Source: three-view drawing plus pictorial views. Frame: mm from the lowest corner of the part. Give positions to 0.01 mm unless a question says otherwise; leave off trailing zeros. Loops run counter-clockwise (first coordinate to the right, second up) from the corner with the lowest first, then second, coordinate; pieces in that order, holes last. Notation, with made-up numbers: (50, 52) - (101, 52) arc R26 ccw to (101, 91) - close; hole circle Ø8 at (-15.5, -32). An arc over 180 degrees is marked (long way). Answer as a JSON object with one key per item and string values. Group by question number.
(1) Section query B-B (y = 4.3). Return loops of the section in (x, z), plus the area to 3 significant figures.
(2) Material intervals for L1, parallel to X at y = 0.3, z = 2.9; L2, parallel to Z at x = 55, y = 3.1; L3, parallel to Y at x = 57, z = 4.1, sorted ascending.
(3) Mould query, pull axis X, two halves, no side actions, for the marked faces 1, 2, 3 and 4. Classes: +X half, -X half, draft (parallel to the pull), parting line (faces both ways), or undercut.
(4) Pin query (flat end, axial travel): P1, Ø3.5, axis at x = 14.5, z = 3.5, coming from the +Y side. Return the tip coordinate at first contact, or that it passes through.
(5) Section query D-D (y = 2.1). Return loops of the section in (x, z).
(6) Section query C-C (x = 53.5). Return loops of the section in (y, z), plus the area to 3 significant figures.
(7) Section query A-A (z = 3). Return loops of the section in (x, y), plus the area to 3 significant figures.
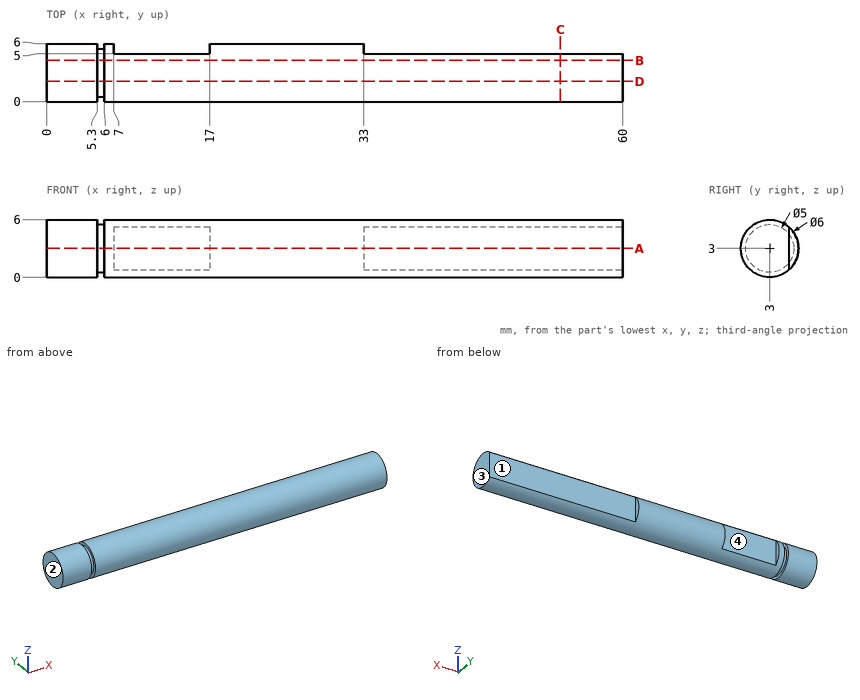
Recorded:
{
 "1": {"outline": "(0, 0.3) - (5.3, 0.3) - (5.3, 0.86) - (6, 0.86) - (6, 0.3) - (60, 0.3) - (60, 5.7) - (6, 5.7) - (6, 5.14) - (5.3, 5.14) - (5.3, 5.7) - (0, 5.7) - close", "area": "324 mm^2"},
 "2": {"L1": "x = 0 to 5.3, 6 to 60", "L2": "z = 0 to 6", "L3": "y = 0.21 to 5"},
 "3": {"face 1": "draft", "face 2": "-X half", "face 3": "+X half", "face 4": "undercut"},
 "4": {"P1": "stops at y = 5"},
 "5": {"outline": "(0, 0.14) - (5.3, 0.14) - (5.3, 0.67) - (6, 0.67) - (6, 0.14) - (60, 0.14) - (60, 5.86) - (6, 5.86) - (6, 5.33) - (5.3, 5.33) - (5.3, 5.86) - (0, 5.86) - close"},
 "6": {"outline": "(5, 0.76) - (5, 5.24) arc R3 ccw (long way) to start", "area": "25.2 mm^2"},
 "7": {"outline": "(0, 0) - (5.3, 0) - (5.3, 0.5) - (6, 0.5) - (6, 0) - (60, 0) - (60, 5) - (33, 5) - (33, 6) - (17, 6) - (17, 5) - (7, 5) - (7, 6) - (6, 6) - (6, 5.5) - (5.3, 5.5) - (5.3, 6) - (0, 6) - close", "area": "322 mm^2"}
}
